Could you check a few things on this model? Use its own coordinates, in mm. Face numbers are marked on the shaded views. A direction names the side the tool comes from. Give positions to 0.01 mm unless a question says otherwise; leave off trailing zeros. Loops run counter-clockwise (first coordinate to the right, second up) from the corner with the lowest first, then second, coordinate; pieces in that order, holes last. Notation, with made-up numbers: (-21, 23) -> (14, 23) arc R30 ccw to (14, 49) -> close; hole circle Ø11 at (-35, 21). An arc over 180 degrees is marked (long way). Write each question's results on one line, items separated by ' | '. Start each with the question number.
Q1. Will these pins go through, and if not, where does the flat tip stop? P1, Ø2, axis at x = 66.5, z = -135.5, coming from the -Y side; P2, Ø8, axis at x = 72, z = -68.5, coming from the +Y side; P3, Ø12, axis at x = 94, z = 49, coming from the -Y side.
Q2. If we section it at C-C, the plane z = 206: List the corners of the cut face in (x, y) for me.
Q3. If we section it at D-D, the plane y = -200: List the corners of the cut face in (x, z) for me.
Q4. If we section it at A-A, the plane y = 0: Give the number of separate pieces and of enclosed holes in the cut face, plus the area to 3 significant figures.
Q5. We'd pull the mould along Z, two halves only. Please class the marked faces 3, 4 and 5: released by +Z, released by -Z, zero draft, split by the parting line, or undercut.
Q6. Which directions (+Z, -Z, +X, -X, +Y, -Y) give clear straight access to the entire face, cutting with the end or side of a thin tool? Please do the marked faces 1 and 2.
Q7. If I drill on line 1 along Z through (x, y) = (15, 0); line 2 along Y through (x, z) = (8, -176); line 3 along Y through (x, z) = (42.5, 37), over which ranges is the centre line in solid material (lowest first)?
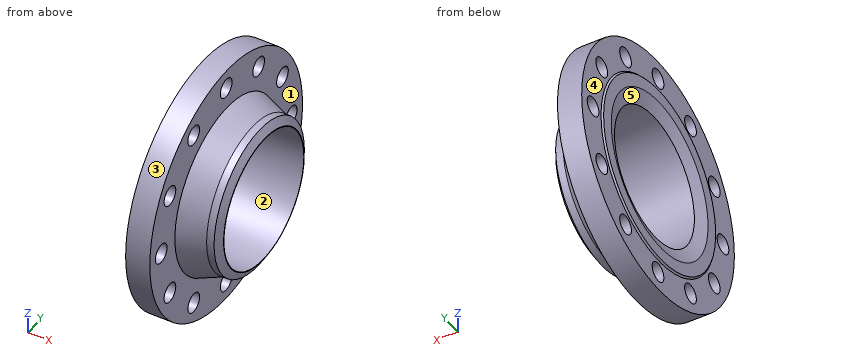
Autodesk Inventor part; units mm, degrees
ref_plane "YZ Plane" through (0, 0, 0) normal (1, 0, 0) x (0, 1, 0)
ref_plane "XZ Plane" through (0, 0, 0) normal (0, 1, 0) x (-1, 0, 0)
ref_plane "XY Plane" through (0, 0, 0) normal (0, 0, 1) x (1, 0, 0)
sketch "Sketch1" plane through (0, 0, 0) normal (0, 0, 1) x (1, 0, 0)
  line L0 (3, 235) -> (48, 235)
  line L1 (48, 235) -> (48, 158)
  line L2 (3, 175.5) -> (3, 235)
  line L3 (-23.6, 0) -> (141.6, 0)
  line L4 (48, 158) -> (95.5, 139)
  line L5 (95.5, 139) -> (109.3397, 139)
  line L6 (118, 124) -> (118, 123)
  line L7 (118, 123) -> (9.721, 123)
  line L8 (3, 175.5) -> (0, 172.5)
  line L9 (0, 172.5) -> (0, 149)
  line L10 (118, 124) -> (109.3397, 139)
  line L11 (9.721, 123) -> (0, 149)
  point P0 (0, 0)
  point P1 (118, 139)
  dimension "d0" = 45
  dimension "d1" = 470
  dimension "d7" = 246
  dimension "d8" = 345
  dimension "d9" = 316
  dimension "d10" = 135
  dimension "d11" = 3
  dimension "d19" = 19
  dimension "d12" = 47.5
  dimension "d13" = 278
  dimension "d14" = 115
  dimension "d15" = 30
  dimension "d16" = 1
  dimension "d17" = 20.5
  dimension "d18" = 298
revolve "Revolution1" add sketch "Sketch1" angle 360 about axis through (-10, 0, 0) along (1, 0, 0)
sketch "Sketch2" plane through (0, 0, 0) normal (1, 0, 0) x (0, 1, 0)
  circle A0 centre (0, 200) radius 18
  line L0 (0, 44.8) -> (0, 25.2) construction
  line L1 (-9.8, 0) -> (9.8, 0) construction
  dimension "d2" = 36
  dimension "d3" = 400
extrude "Extrusion1" cut sketch "Sketch2" along normal through all both and the other way through all
pattern_circular "Circular Pattern1" count 12 over 360 about axis through (-10, 0, 0) along (1, 0, 0) of "Extrusion1"
equation "\"d2\" = d"
equation "\"d3\" = D1_"
equation "\"d0\" = b"
equation "\"d1\" = D_"
equation "\"d7\" = d1__"
equation "\"d8\" = D2_"
equation "\"d9\" = Dm"
equation "\"d11\" = h_"
equation "\"d12\" = 2.5 * d19"
equation "\"d13\" = Dn"
equation "\"d14\" = h4_"
equation "\"d18\" = D7_"
equation "\"b\" = 45"
equation "\"Dm\" = 316"
equation "\"D_\" = 470"
equation "\"D1_\" = 400"
equation "\"D2_\" = 345"
equation "\"d\" = 36"
equation "\"h_\" = 3"
equation "\"d1__\" = 246"
equation "\"h4_\" = 115"
equation "\"Dn\" = 278"
equation "\"D7_\" = 298"
properties part number "Flange 6-250-63-1 GOST 12821-80" material "Steel, Mild"
Final values:
1) P1: stops at y = -67.94 | P2: stops at y = 134.34 | P3: stops at y = -134.04
2) outline: (3, -113.09) -> (48, -113.09) -> (48, -16.97) -> (3, -16.97) -> close; (3, 16.97) -> (48, 16.97) -> (48, 113.09) -> (3, 113.09) -> close
3) outline: (3, -123.39) -> (48, -123.39) -> (48, -18) -> (3, -18) -> close; (3, 18) -> (48, 18) -> (48, 123.39) -> (3, 123.39) -> close
4) separate pieces: 4 | enclosed holes: 0 | area: 9,910 mm²
5) face 3: split by the parting line | face 4: zero draft | face 5: undercut
6) face 1: +X | face 2: +X, -X
7) line 1: z = -235 to -218, -182 to -123, 123 to 182, 218 to 235 | line 2: y = -155.72 to -117.78, -82.22 to 82.22, 117.78 to 155.72 | line 3: y = -232.07 to -117.3, 117.3 to 232.07
